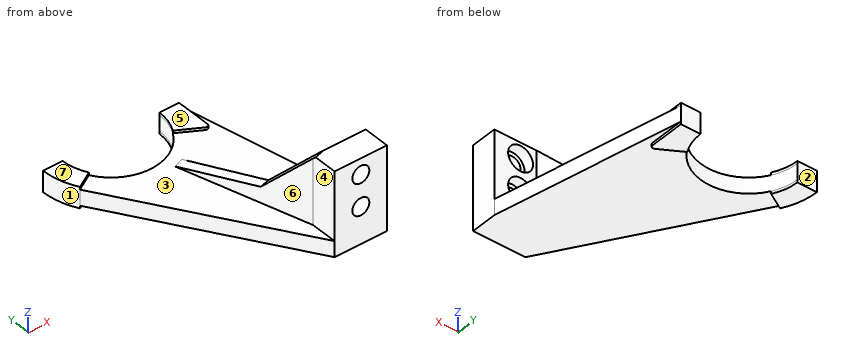
from build123d import *

# Parameters (mm, degrees)
SALIENTE_EXTRUIR1_DEPTH = 9.525
CROQUIS2_W              = 31.75
CROQUIS2_H              = 15.875
SALIENTE_EXTRUIR2_DEPTH = 41.275
CROQUIS3_R              = 5.159375
CORTAR_EXTRUIR1_DEPTH   = 133.943055
CROQUIS4_R              = 7.540625
CORTAR_EXTRUIR2_DEPTH   = 6.35
SALIENTE_EXTRUIR5_DEPTH = 6.35
REDONDEO1_R             = 1.5875
REDONDEO4_R             = 1.5875
SALIENTE_EXTRUIR8_DEPTH = 41.275
CORTAR_EXTRUIR4_DEPTH   = 41.275


with BuildPart() as part:
    # Croquis1 → Saliente-Extruir1 (new body)
    with BuildSketch(Plane.XY):
        with BuildLine():
            Line((-52.3875, 63.5), (-40.48125, 63.5))
            ThreePointArc((-40.48125, 63.5), (-11.1125, 34.13125), (18.25625, 63.5))
            Line((18.25625, 63.5), (30.1625, 63.5))
            Line((30.1625, 63.5), (52.3875, -47.625))
            Line((52.3875, -47.625), (52.3875, -63.5))
            Line((52.3875, -63.5), (20.6375, -63.5))
            Line((20.6375, -63.5), (-46.857699, 42.8625))
            ThreePointArc((-46.857699, 42.8625), (-50.981088, 52.817244), (-52.3875, 63.5))
        make_face()
    extrude(amount=SALIENTE_EXTRUIR1_DEPTH)

    # Croquis2 → Saliente-Extruir2 (add)
    with BuildSketch(Plane.XY.offset(9.525)):
        with Locations((36.5125, -55.5625)):
            Rectangle(CROQUIS2_W, CROQUIS2_H)
    extrude(amount=SALIENTE_EXTRUIR2_DEPTH)

    # Croquis3 → Cortar-Extruir1 (cut, through all)
    with BuildSketch(Plane(origin=(0, -47.625, 0), x_dir=(1, 0, 0), z_dir=(0, 1, 0))):
        with Locations(Location((36.5125, -41.275, 0), (0, 0, 270))):
            Circle(CROQUIS3_R)
        with Locations(Location((36.5125, -22.225, 0), (0, 0, 270))):
            Circle(CROQUIS3_R)
    extrude(amount=-CORTAR_EXTRUIR1_DEPTH, mode=Mode.SUBTRACT)

    # Croquis4 → Cortar-Extruir2 (cut)
    with BuildSketch(Plane(origin=(0, -47.625, 0), x_dir=(1, 0, 0), z_dir=(0, 1, 0))):
        with Locations(Location((36.5125, -22.225, 0), (0, 0, 270))):
            Circle(CROQUIS4_R)
        with Locations(Location((36.5125, -41.275, 0), (0, 0, 270))):
            Circle(CROQUIS4_R)
    extrude(amount=-CORTAR_EXTRUIR2_DEPTH, mode=Mode.SUBTRACT)

    # Croquis8 → Saliente-Extruir5 (add, symmetric)
    with BuildSketch(Plane.XY.offset(4.7625)):
        with BuildLine():
            Line((-52.3875, 63.5), (-40.48125, 63.5))
            ThreePointArc((-40.48125, 63.5), (-39.480534, 55.898808), (-36.546584, 48.815625))
            Line((-36.546584, 48.815625), (-46.857699, 42.8625))
            ThreePointArc((-46.857699, 42.8625), (-50.981088, 52.817244), (-52.3875, 63.5))
        make_face()
        with BuildLine():
            ThreePointArc((14.321584, 48.815625), (17.255534, 55.898808), (18.25625, 63.5))
            Line((18.25625, 63.5), (30.1625, 63.5))
            Line((30.1625, 63.5), (30.1625, 39.669868))
            Line((30.1625, 39.669868), (14.321584, 48.815625))
        make_face()
    extrude(amount=SALIENTE_EXTRUIR5_DEPTH, both=True)

    # Redondeo1
    redondeo1_edges = [part.edges().sort_by_distance(p)[0] for p in [
        (30.1625, 39.669868, 10.31875),
    ]]
    fillet(redondeo1_edges, radius=REDONDEO1_R)

    # Redondeo4
    redondeo4_edges = [part.edges().sort_by_distance(p)[0] for p in [
        (30.1625, 39.669868, -0.79375),
    ]]
    fillet(redondeo4_edges, radius=REDONDEO4_R)

    # Croquis9 → Saliente-Extruir8 (add)
    with BuildSketch(Plane.XY.offset(9.525)):
        Polygon((-0.982547, 28.253318), (20.6375, -47.625), (23.8125, -47.625), (26.9875, -47.625), (4.929446, 30.570825), (1.97345, 29.412071), align=None)
    extrude(amount=SALIENTE_EXTRUIR8_DEPTH)

    # Croquis12 → Cortar-Extruir4 (cut)
    with BuildSketch(Plane(origin=(12.554117, 3.541358, 0), x_dir=(0, 0, -1), z_dir=(0.9624406031715071, 0.27149233021738517, 0))):
        Polygon((-9.525, 28.084296), (-50.8, 28.084296), (-50.8, -53.163133), (-19.05, -21.413133), align=None)
    extrude(amount=-CORTAR_EXTRUIR4_DEPTH, mode=Mode.SUBTRACT)


solid = part.part
Design review of the part built by this model. Coordinates are the model's own, in mm. Face numbers are marked on the shaded views. A direction names the side the tool comes from. Give positions to 0.01 mm unless a question says otherwise; leave off trailing zeros. Loops run counter-clockwise (first coordinate to the right, second up) from the corner with the lowest first, then second, coordinate; pieces in that order, holes last. Notation, with made-up numbers: (16, 57) - (51, 57) arc R11 ccw to (51, 68) - close; hole circle Ø7 at (41.5, 85.5). An arc over 180 degrees is marked (long way). Write item = value, one per line.
1) Tool access review of the marked faces 5, 6 and 7: name each direction out of +Z, -Z, +X, -X, +Y, -Y from which nothing blocks a thin tool from reaching the whole face with its end or side.
Result sheet:
face_5 = +Z, +X, -X, +Y
face_6 = +Z, -X, -Y
face_7 = +Z, +X, -X, +Y, -Y
2) Take a section at C-C on z = 42.5. State the section outline as (x, y) points (1 decimal), and give its area (3 significant figures).
Result sheet:
outline = (18.8, -41.3) - (20.6, -47.6) - (20.6, -63.5) - (31.5, -63.5) - (31.5, -54) - (29.1, -54) - (29.1, -47.6) - (27, -47.6) - (24.7, -39.6) - close; (41.5, -63.5) - (52.4, -63.5) - (52.4, -47.6) - (44, -47.6) - (44, -54) - (41.5, -54) - close
area = 360 mm2
3) Take a section at B-B on y = -3.5. State the section outline as (x, z) points (1 decimal).
Result sheet:
outline = (-17.4, 0) - (43.6, 0) - (43.6, 9.5) - (14.5, 9.5) - (14.5, 16.3) - (8.1, 16) - (8.1, 9.5) - (-17.4, 9.5) - close
4) Take a section at A-A on z = 24.5. State the section outline as (x, y) points (1 decimal), and give its area (3 significant figures).
Result sheet:
outline = (13.9, -24) - (20.6, -47.6) - (20.6, -63.5) - (31.9, -63.5) - (31.9, -54) - (29.3, -54) - (29.3, -47.6) - (27, -47.6) - (19.8, -22.3) - close; (41.1, -63.5) - (52.4, -63.5) - (52.4, -47.6) - (43.7, -47.6) - (43.7, -54) - (41.1, -54) - close
area = 481 mm2
5) Draft analysis for pull direction Y (two halves, no side actions). For the marked faces 1, 2, 3 and 4, state which applies: +Y half, -Y half, draft (parallel to the pull), parting line (faces both ways), or undercut.
Result sheet:
face_1 = -Y half
face_2 = +Y half
face_3 = undercut
face_4 = draft
6) To check wall thickness, follow line 1 (Z direction, x = 13.5, y = 39) (3 decimals); line 2 (Y direction, x = 8.5, z = 3.5); line 3 (Y direction, x = 7, z = 5). State the ranges of each line that lie inside material, in increasing order.
Result sheet:
line_1 = 0 to 9.525
line_2 = -44.37 to 41.64
line_3 = -42.01 to 40.38
7) Clearance check with flat-ended pins moving along their axes: pin 1 Ø12.5 at (x, y) = (19, 57.5) entering from +Z; pin 2 Ø12 at (x, z) = (37, 39) entering from +Y (3 decimals); pin 3 Ø12 at (x, z) = (11.5, 26) entering from +Y; pin 4 Ø8 at (y, z) = (27, 16.5) entering from -X. State where each tip first meets the part, or that it passes through.
Result sheet:
pin_1 = 11.11
pin_2 = -47.625
pin_3 = -19.77
pin_4 = through
